Here's the drawing with two shaded views (mm, measured from the low corner). I have some questions. Round coordinates to 2 decimals unless told otherwise and drop trailing zeros. One line per item, written item: value. Start each with the question number.
Q1. Imagine slicing it at A-A (x = 8.25). Give the number of separate pieces and of enclosed holes in the cut face, then the cut area to 3 significant figures.
Q2. I'm going to push flat-ended pins straight in: pin 1 Ø15 at (y, z) = (34.41, 47.05) entering from +X (3 decimals); pin 2 Ø5 at (x, z) = (6.5, 28.5) entering from -Y; pin 3 Ø5 at (x, z) = (9.5, 131) entering from -Y; pin 4 Ø4 at (x, z) = (13, 77) entering from -Y. Where does each tip first touch, or does it pass through?
Q3. Please list where these lines run through material, in increasing order: line 1 along Z through (x, y) = (11.25, 63.5) (1 decimal); line 2 along Y through (x, z) = (2.25, 85.5) (1 decimal); line 3 along Z through (x, y) = (12.25, 32) (1 decimal).
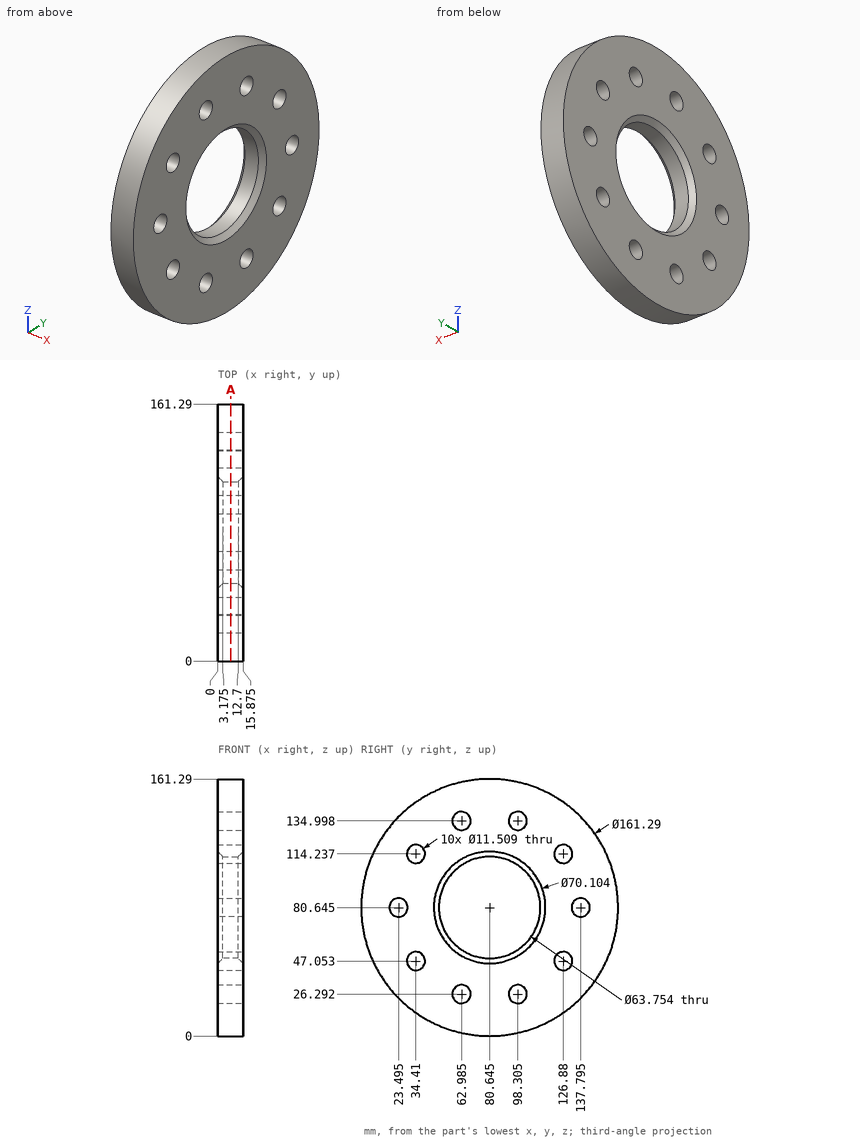
Report:
1. separate pieces: 1
1. enclosed holes: 11
1. area: 16,200 mm²
2. pin 1: stops at x = 15.875
2. pin 2: stops at y = 17.09
2. pin 3: stops at y = 15.73
2. pin 4: stops at y = 0.02
3. line 1: z = 1.8 to 20.6, 32 to 53.8, 107.5 to 129.3, 140.7 to 159.4
3. line 2: y = 0.1 to 20.4, 26.6 to 48.2, 113.1 to 134.7, 140.9 to 161.1
3. line 3: z = 16.3 to 41.8, 52.3 to 109, 119.5 to 145
